from build123d import *

# Parameters (mm, degrees)
F0_W     = 0.5
F0_H     = 3.5
F0_R     = 1.25
F1_DEPTH = 4.3564048
F2_R     = 0.762
F3_W     = 19.038
F3_H     = 6.3
F3_H_2   = 3.5
F4_DEPTH = 4.3564048


with BuildPart() as f1:
    # F0 (on Top) → F1 (new body)
    with BuildSketch(Plane.XY):
        with Locations((4.1668843009, -11.25)):
            Rectangle(F0_W, F0_H)
        with Locations((-3.3831156991, -11.25)):
            Rectangle(F0_W, F0_H)
        with Locations((-11.9331156991, -11.25)):
            Rectangle(F0_W, F0_H)
        with BuildLine():
            Line((-10.6081156991, 0.7), (-9.8143656991, 0.7))
            Line((-9.8143656991, 0.7), (-9.8143656991, 1.101979753))
            ThreePointArc((-9.8143656991, 1.101979753), (-9.7252470071, 1.317131308), (-9.5100954521, 1.40625))
            Line((-9.5100954521, 1.40625), (6.0168843009, 1.40625))
            Line((6.0168843009, 1.40625), (6.0168843009, 2.2))
            Line((6.0168843009, 2.2), (6.0168843009, 4.6))
            ThreePointArc((6.0168843009, 4.6), (3.6168843009, 7), (1.2168843009, 4.6))
            Line((1.2168843009, 4.6), (1.2168843009, 2.2))
            Line((1.2168843009, 2.2), (-9.5100954521, 2.2))
            ThreePointArc((-9.5100954521, 2.2), (-10.2865130147, 1.8783973155), (-10.6081156991, 1.101979753))
            Line((-10.6081156991, 1.101979753), (-10.6081156991, 0.7))
        make_face()
        with BuildLine():
            Line((6.0168843009, 0), (0, 0))
            Line((0, 0), (-0.7, 0.7))
            Line((-0.7, 0.7), (-5.9126656991, 0.7))
            ThreePointArc((-5.9126656991, 0.7), (-6.5935156991, 1.38085), (-7.2743656991, 0.7))
            Line((-7.2743656991, 0.7), (-9.8143656991, 0.7))
            Line((-9.8143656991, 0.7), (-10.6081156991, 0.7))
            Line((-10.6081156991, 0.7), (-13.7831156991, 0.7))
            Line((-13.7831156991, 0.7), (-13.7831156991, -9.5))
            Line((-13.7831156991, -9.5), (-12.1831156991, -9.5))
            Line((-12.1831156991, -9.5), (-11.6831156991, -9.5))
            Line((-11.6831156991, -9.5), (-3.6331156991, -9.5))
            Line((-3.6331156991, -9.5), (-3.1331156991, -9.5))
            Line((-3.1331156991, -9.5), (3.9168843009, -9.5))
            Line((3.9168843009, -9.5), (4.4168843009, -9.5))
            Line((4.4168843009, -9.5), (6.0168843009, -9.5))
            Line((6.0168843009, -9.5), (6.0168843009, 0))
        make_face()
        with Locations((-8.6831156991, -6.6)):
            Circle(F0_R, mode=Mode.SUBTRACT)
        with Locations((0.8168843009, -6.6)):
            Circle(F0_R, mode=Mode.SUBTRACT)
    extrude(amount=F1_DEPTH)

    # F2
    f2_edges = [f1.edges().sort_by_distance(p)[0] for p in [
        (6.016884, 0, 2.178202),
        (-13.783116, -9.5, 2.178202),
        (-13.783116, 0.7, 2.178202),
    ]]
    fillet(f2_edges, radius=F2_R)

    # F3 (on face) → F4 (cut, through all)
    with BuildSketch(Plane.XY.offset(4.3564048)):
        with Locations((-3.5021156991, 3.85)):
            Rectangle(F3_W, F3_H)
        with Locations((-3.5021156991, -11.25)):
            Rectangle(F3_W, F3_H_2)
    extrude(amount=-F4_DEPTH, mode=Mode.SUBTRACT)


solid = f1.part
Work out the finished part from the listing and answer in its coordinate system (mm). A direction names the side the tool comes from. Round coordinates to 2 decimals unless told otherwise and drop trailing zeros. Loops run counter-clockwise (first coordinate to the right, second up) from the corner with the lowest first, then second, coordinate; pieces in that order, holes last. Notation, with made-up numbers: (42.5, 5.25) - (65.5, 5.25) arc R28 ccw to (65.5, 38.25) - close; hole circle Ø4 at (81.25, -9.75). An arc over 180 degrees is marked (long way). One line per item, written item: value.
Q1. For faces 1 (the flat face through (3, 0, 2)), 2 (the cylindrical face through (0.65, -5.36, 2.15)), determine the directions among +Z, -Z, +X, -X, +Y, -Y from which every point of the face is accessible in a straight line to the end or side of a thin tool.
Check values:
face 1: +Z, -Z, +X, +Y
face 2: +Z, -Z
Q2. Find section A-A on y = -6.6. Give the vertices of the cut face in (x, z), and give its area (3 significant figures).
Check values:
outline: (-13.78, 0) - (-9.93, 0) - (-9.93, 4.36) - (-13.78, 4.36) - close; (-7.43, 0) - (-0.43, 0) - (-0.43, 4.36) - (-7.43, 4.36) - close; (2.07, 0) - (6.02, 0) - (6.02, 4.36) - (2.07, 4.36) - close
area: 64.5 mm2
Q3. The mould has two halves that part along X. Classify faces 3 (the flat face through (-4, -4, 0)), 4 (the flat face through (-13.783, -4, 2)), 5 (the flat face through (6.017, -5, 2)), 6 (the cylindrical face through (-7.5, -6.2, 2.1)): +X half, -X half, draft (parallel to the pull), parting line (faces both ways), or undercut.
Check values:
face 3: draft
face 4: -X half
face 5: +X half
face 6: undercut
Q4. Find section C-C on x = 0.5. Give the vertices of the cut face in (y, z).
Check values:
outline: (-9.5, 0) - (-7.81, 0) - (-7.81, 4.36) - (-9.5, 4.36) - close; (-5.39, 0) - (0, 0) - (0, 4.36) - (-5.39, 4.36) - close
Q5. Straight lines are drawn through the part: probe 1 along Y at (x, z) = (2.5, 3.2); probe 2 along Y at (x, z) = (1.5, 2.7); probe 3 along Y at (x, z) = (-9.75, 1.2). For each, find the intervals that lie inside material, in ascending order.
Check values:
probe 1: -9.5 to 0
probe 2: -9.5 to -7.65, -5.55 to 0
probe 3: -9.5 to -7.25, -5.95 to 0.7
Q6. Find section B-B on z = 1.55. Give the vertices of the cut face in (x, y).
Check values:
outline: (-13.78, -8.74) arc R0.76 ccw to (-13.02, -9.5) - (6.02, -9.5) - (6.02, -0.76) arc R0.76 ccw to (5.25, 0) - (0, 0) - (-0.7, 0.7) - (-13.02, 0.7) arc R0.76 ccw to (-13.78, -0.06) - close; hole circle Ø2.5 at (-8.68, -6.6); hole circle Ø2.5 at (0.82, -6.6)
Q7. This flat-tipped pin is pushed along its axis until it touches: pin 1 Ø2 at (x, z) = (2.5, 2.5) entering from +Y. Where does it stop, or does it pass through?
Check values:
pin 1: y = 0
